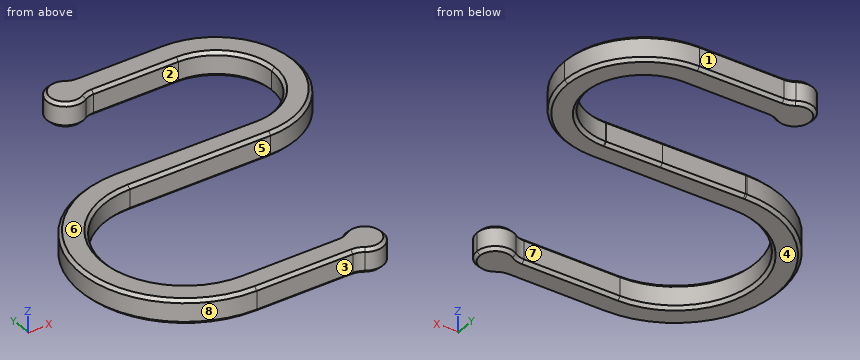
from build123d import *

# Parameters (mm, degrees)
F1_DEPTH = 4
F2_R     = 3
F3_SIZE  = 0.5


with BuildPart() as f1:
    # F0 (on Top) → F1 (new body)
    with BuildSketch(Plane.XY):
        with BuildLine():
            Line((0.2956298201, 16.9974293059), (0, 17))
            ThreePointArc((0, 17), (-17, 0), (0, -17))
            ThreePointArc((0, -17), (5.8309518948, -15.9687194227), (10.9544511501, -13))
            Line((10.9544511501, -13), (0, -13))
            ThreePointArc((0, -13), (-13, 0), (0, 13))
            Line((0, 13), (10.9544511501, 13))
            ThreePointArc((10.9544511501, 13), (5.9695846357, 15.9174137119), (0.2956298201, 16.9974293059))
        make_face()
        with BuildLine():
            ThreePointArc((10.9544511501, -13), (5.8309518948, -15.9687194227), (0, -17))
            Line((0, -17), (16.7639320225, -17))
            ThreePointArc((16.7639320225, -17), (16, -15), (16.7639320225, -13))
            Line((16.7639320225, -13), (10.9544511501, -13))
        make_face()
        with BuildLine():
            Line((13.73523492, 16.8805631746), (0.2956298201, 16.9974293059))
            ThreePointArc((0.2956298201, 16.9974293059), (5.9695846357, 15.9174137119), (10.9544511501, 13))
            Line((10.9544511501, 13), (23, 13))
            ThreePointArc((23, 13), (17.9776837381, 14.0093228146), (13.73523492, 16.8805631746))
        make_face()
        with BuildLine():
            ThreePointArc((16.7639320225, -13), (16, -15), (16.7639320225, -17))
            Line((16.7639320225, -17), (19, -17))
            Line((19, -17), (19, -13))
            Line((19, -13), (16.7639320225, -13))
        make_face()
        with BuildLine():
            Line((19, -17), (16.7639320225, -17))
            ThreePointArc((16.7639320225, -17), (20.0704662693, -17.8025170769), (22, -15))
            ThreePointArc((22, -15), (20.0704662693, -12.1974829231), (16.7639320225, -13))
            Line((16.7639320225, -13), (19, -13))
            Line((19, -13), (19, -17))
        make_face()
        with BuildLine():
            Line((22.8434900953, 16.8013609557), (13.73523492, 16.8805631746))
            ThreePointArc((13.73523492, 16.8805631746), (17.9776837381, 14.0093228146), (23, 13))
            ThreePointArc((23, 13), (32.1923881554, 16.8076118446), (36, 26))
            ThreePointArc((36, 26), (32.1923881554, 35.1923881554), (23, 39))
            ThreePointArc((23, 39), (17.775059809, 37.903780912), (13.4313010289, 34.8))
            Line((13.4313010289, 34.8), (23, 34.8))
            ThreePointArc((23, 34.8), (29.3639610307, 32.1639610307), (32, 25.8))
            ThreePointArc((32, 25.8), (29.3639610307, 19.4360389693), (23, 16.8))
            ThreePointArc((23, 16.8), (22.9217420891, 16.8003402454), (22.8434900953, 16.8013609557))
        make_face()
        with BuildLine():
            Line((8.1424285286, 34.8), (13.4313010289, 34.8))
            ThreePointArc((13.4313010289, 34.8), (17.775059809, 37.903780912), (23, 39))
            Line((23, 39), (8.1424285286, 39))
            ThreePointArc((8.1424285286, 39), (8.7773445578, 38.0341768853), (9, 36.9))
            ThreePointArc((9, 36.9), (8.7773445578, 35.7658231147), (8.1424285286, 34.8))
        make_face()
        with BuildLine():
            ThreePointArc((8.1424285286, 39), (3, 36.9), (8.1424285286, 34.8))
            Line((8.1424285286, 34.8), (6, 34.8))
            Line((6, 34.8), (6, 39))
            Line((6, 39), (8.1424285286, 39))
        make_face()
        with BuildLine():
            Line((6, 34.8), (8.1424285286, 34.8))
            ThreePointArc((8.1424285286, 34.8), (8.7773445578, 35.7658231147), (9, 36.9))
            ThreePointArc((9, 36.9), (8.7773445578, 38.0341768853), (8.1424285286, 39))
            Line((8.1424285286, 39), (6, 39))
            Line((6, 39), (6, 34.8))
        make_face()
    extrude(amount=F1_DEPTH)

    # F2
    f2_edges = [f1.edges().sort_by_distance(p)[0] for p in [
        (16.763932, -17, 2),
        (8.142429, 34.8, 2),
        (16.763932, -13, 2),
        (8.142429, 39, 2),
    ]]
    fillet(f2_edges, radius=F2_R)

    # F3
    f3_edges = [f1.edges().sort_by_distance(p)[0] for p in [
        (7.841688, -17, 4),
        (7.841688, -13, 4),
        (-13, 0, 4),
        (-17, 0, 4),
        (11.5, 13, 4),
        (11.421745, 16.90068, 4),
        (22, -15, 4),
        (16.549401, -12.872281, 4),
        (16.549401, -17.127719, 4),
        (36, 26, 4),
        (31.99966, 25.721742, 4),
        (16.080348, 34.8, 4),
        (16.080348, 39, 4),
        (8.339112, 34.685308, 4),
        (8.339112, 39.114692, 4),
        (3, 36.9, 4),
        (22, -15, 0),
        (16.549401, -17.127719, 0),
        (7.841688, -13, 0),
        (7.841688, -17, 0),
        (16.549401, -12.872281, 0),
        (-13, 0, 0),
        (-17, 0, 0),
        (11.5, 13, 0),
        (11.421745, 16.90068, 0),
        (31.99966, 25.721742, 0),
        (16.080348, 34.8, 0),
        (8.339112, 34.685308, 0),
        (3, 36.9, 0),
        (36, 26, 0),
        (8.339112, 39.114692, 0),
        (16.080348, 39, 0),
    ]]
    chamfer(f3_edges, length=F3_SIZE)


solid = f1.part
Can you work these out from the model? Positions are in its coordinate system, mm. Face numbers are marked on the shaded views. A direction names the side the tool comes from. Give positions to 0.01 mm unless a question says otherwise; leave off trailing zeros. Loops run counter-clockwise (first coordinate to the right, second up) from the corner with the lowest first, then second, coordinate; pieces in that order, holes last. Notation, with made-up numbers: M 85.25,62.5 L 91.25,62.5 A17 cw 91.25,87.5 Z; hole C 78.25,33 d5. An arc over 180 degrees is marked long. One line per item, written item: value. Start each with the question number.
1) If we section it at C-C, the plane x = 6: Write out the boundary of the cut face in (y, z), and give its area (3 significant figures).
2) If we section it at A-A, the plane z = 1.2: Write out the boundary of the cut face in (x, y), and give its area (3 significant figures).
3) If we section it at B-B, the plane y = 0: Write out the boundary of the cut face in (x, z), and give its area (3 significant figures).
4) Thinking about a two-plate mould opening in X: for the marked faces 6, 7 and 8, which applies, +X half, -X half, draft (parallel to the pull), parting line (faces both ways), or undercut?
5) On a 3-axis mill with a long thin cutter (end or side, diameter ignored), from which of +Z, -Z, +X, -X, +Y, -Y can I reach the whole of each face in a straight line? I mean the marked faces 1, 2, 3, 4 and 5. Say none if no direction works.
6) I'm going to push flat-ended pins straight in: pin 1 (1.5 mm diameter, centred on x = 18, z = 2.5, fed in from +Y); pin 2 (0.9 mm diameter, centred on x = 15, z = 2.5, fed in from -Y); pin 3 (1 mm diameter, centred on x = 29.5, z = 2, fed in from +Y). Where does each tip first touch, or does it pass through?
7) If I drill on line 1 (Y direction, x = 6.5, z = 2.4); line 2 (Y direction, x = 4, z = 3.6); line 3 (Y direction, x = 24, z = 3.6), over which ranges is the centre line in solid material (lowest first)? Write a range as [from, to].
Completed:
1. outline: M -17,0.5 L -16.5,0 L -13.5,0 L -13,0.5 L -13,3.5 L -13.5,4 L -16.5,4 L -17,3.5 Z; M 13,0.5 L 13.5,0 L 16.45,0 L 16.95,0.5 L 16.95,3.5 L 16.45,4 L 13.5,4 L 13,3.5 Z; M 33.9,0.5 L 34.4,0 L 39.4,0 L 39.9,0.5 L 39.9,3.5 L 39.4,4 L 34.4,4 L 33.9,3.5 Z
1. area: 54.3 mm^2
2. outline: M 0,-17 L 15.68,-17 A3 cw 17.34,-17.5 A3 ccw long 17.34,-12.5 A3 cw 15.68,-13 L 0,-13 A13 cw 0,13 L 23,13 A13 ccw 23,39 L 9.16,39 A3 cw 7.58,39.45 A3 ccw long 7.58,34.35 A3 cw 9.16,34.8 L 23,34.8 A9 cw 23,16.8 A9 cw 22.84,16.8 L 0,17 A17 ccw Z
2. area: 598 mm^2
3. outline: M -17,0.5 L -16.5,0 L -13.5,0 L -13,0.5 L -13,3.5 L -13.5,4 L -16.5,4 L -17,3.5 Z
3. area: 15.5 mm^2
4. face 6: draft
4. face 7: undercut
4. face 8: -X half
5. face 1: +Z, -Z, +X, +Y
5. face 2: +Z, -Z
5. face 3: +Z, -Z, -X, -Y
5. face 4: -Z, +X, -X, +Y, -Y
5. face 5: +Z, -Z, +X
6. pin 1: stops at y = 39
6. pin 2: stops at y = -17
6. pin 3: stops at y = 37.53
7. line 1: y = [-17, -13], [13, 16.94], [33.94, 39.86]
7. line 2: y = [-16.9, -13.1], [13.1, 16.87], [34.8, 39]
7. line 3: y = [13.14, 16.76], [34.84, 38.86]
